from build123d import *

# Parameters (mm, degrees)
SKETCH_1_W                  = 180
SKETCH_1_H                  = 160
EXTRUDE_1_DEPTH             = 4
SKETCH_4_R                  = 1.6
CUT_EXTRUDE_3_DEPTH         = 4
SKETCH_5_R                  = 1.6
CUT_EXTRUDE_4_DEPTH         = 4
SKETCH_7_R                  = 2
CUT_EXTRUDE_5_DEPTH         = 10
FILLET_1_R                  = 10
SKETCH_8_R                  = 1.5
CUT_EXTRUDE_6_DEPTH         = 10
SKETCH_11_R                 = 1.5
CUT_EXTRUDE_8_DEPTH         = 4
SKETCH_12_R                 = 1.5
CUT_EXTRUDE_9_DEPTH         = 4
SKETCH_13_R                 = 1.5
CUT_EXTRUDE_10_DEPTH        = 10
PATTERN_LINEAR_1_COUNT      = 2
PATTERN_LINEAR_1_PITCH      = 30
PATTERN_LINEAR_1_COUNT_DIR2 = 2
PATTERN_LINEAR_1_PITCH_DIR2 = 30
MIRROR_1_COPY_1_SKETCH_R    = 1.5
MIRROR_1_COPY_1_DEPTH       = 10
MIRROR_1_COPY_2_SKETCH_R    = 1.5
MIRROR_1_COPY_2_DEPTH       = 10
MIRROR_1_COPY_3_SKETCH_R    = 1.5
MIRROR_1_COPY_3_DEPTH       = 10


with BuildPart() as part:
    # 草图1 → 凸台-拉伸1 (new body)
    with BuildSketch(Plane(origin=(0, 0, 0), x_dir=(1, 0, 0), z_dir=(0, 1, 0))):
        Rectangle(SKETCH_1_W, SKETCH_1_H)
    extrude(amount=EXTRUDE_1_DEPTH)

    # 草图4 → 切除-拉伸3 (cut)
    with BuildSketch(Plane(origin=(0, 4, 0), x_dir=(1, 0, 0), z_dir=(0, 1, 0))):
        with Locations(Location((-80, 56, 0), (0, 0, 270))):
            Circle(SKETCH_4_R)
        with Locations(Location((-43, 56, 0), (0, 0, 270))):
            Circle(SKETCH_4_R)
        with Locations(Location((-43, 19, 0), (0, 0, 270))):
            Circle(SKETCH_4_R)
        with Locations(Location((-80, 19, 0), (0, 0, 270))):
            Circle(SKETCH_4_R)
    extrude(amount=-CUT_EXTRUDE_3_DEPTH, mode=Mode.SUBTRACT)

    # 草图5 → 切除-拉伸4 (cut)
    with BuildSketch(Plane(origin=(0, 4, 0), x_dir=(1, 0, 0), z_dir=(0, 1, 0))):
        with Locations(Location((-78.7, -7.8, 0), (0, 0, 270))):
            Circle(SKETCH_5_R)
        with Locations(Location((-29.2, -23, 0), (0, 0, 270))):
            Circle(SKETCH_5_R)
        with Locations(Location((-29.2, -50.9, 0), (0, 0, 270))):
            Circle(SKETCH_5_R)
        with Locations(Location((-80, -56, 0), (0, 0, 270))):
            Circle(SKETCH_5_R)
        with Locations(Location((-29.2, -5.1, 0), (0, 0, 90))):
            Circle(SKETCH_5_R)
        with Locations(Location((-29.2, -33, 0), (0, 0, 90))):
            Circle(SKETCH_5_R)
        with Locations(Location((-80, 0, 0), (0, 0, 90))):
            Circle(SKETCH_5_R)
        with Locations(Location((-78.7, -48.2, 0), (0, 0, 90))):
            Circle(SKETCH_5_R)
    extrude(amount=-CUT_EXTRUDE_4_DEPTH, mode=Mode.SUBTRACT)

    # 草图7 → 切除-拉伸5 (cut)
    with BuildSketch(Plane.XZ):
        with Locations(Location((24, 35, 0), (0, 0, 270))):
            Circle(SKETCH_7_R)
        with Locations(Location((10, 35, 0), (0, 0, 270))):
            Circle(SKETCH_7_R)
        with Locations(Location((24, 3, 0), (0, 0, 270))):
            Circle(SKETCH_7_R)
        with Locations(Location((10, 3, 0), (0, 0, 270))):
            Circle(SKETCH_7_R)
    extrude(amount=-CUT_EXTRUDE_5_DEPTH, mode=Mode.SUBTRACT)

    # 圆角1
    fillet_1_edges = [part.edges().sort_by_distance(p)[0] for p in [
        (90, 2, 80),
        (-90, 2, 80),
        (-90, 2, -80),
        (90, 2, -80),
    ]]
    fillet(fillet_1_edges, radius=FILLET_1_R)

    # 草图8 → 切除-拉伸6 (cut)
    with BuildSketch(Plane.XZ):
        with Locations(Location((-14.949747468, 4.949747468, 0), (0, 0, 270))):
            Circle(SKETCH_8_R)
        with Locations(Location((-5.050252532, 4.949747468, 0), (0, 0, 270))):
            Circle(SKETCH_8_R)
        with Locations(Location((-14.949747468, -4.949747468, 0), (0, 0, 270))):
            Circle(SKETCH_8_R)
        with Locations(Location((-5.050252532, -4.949747468, 0), (0, 0, 270))):
            Circle(SKETCH_8_R)
    extrude(amount=-CUT_EXTRUDE_6_DEPTH, mode=Mode.SUBTRACT)

    # 草图11 → 切除-拉伸8 (cut)
    with BuildSketch(Plane.XZ):
        with Locations(Location((77, 12, 0), (0, 0, 270))):
            Circle(SKETCH_11_R)
        with Locations(Location((43, 12, 0), (0, 0, 90))):
            Circle(SKETCH_11_R)
        with Locations(Location((77, -12, 0), (0, 0, 90))):
            Circle(SKETCH_11_R)
        with Locations(Location((43, -12, 0), (0, 0, 270))):
            Circle(SKETCH_11_R)
    extrude(amount=-CUT_EXTRUDE_8_DEPTH, mode=Mode.SUBTRACT)

    # 草图12 → 切除-拉伸9 (cut)
    with BuildSketch(Plane.XZ):
        with Locations(Location((-86, 40, 0), (0, 0, 270))):
            Circle(SKETCH_12_R)
        with Locations(Location((-11, 40, 0), (0, 0, 270))):
            Circle(SKETCH_12_R)
        with Locations(Location((-11, -40, 0), (0, 0, 270))):
            Circle(SKETCH_12_R)
        with Locations(Location((-86, -40, 0), (0, 0, 270))):
            Circle(SKETCH_12_R)
    extrude(amount=-CUT_EXTRUDE_9_DEPTH, mode=Mode.SUBTRACT)

    # 草图13 → 切除-拉伸10 (cut)
    with BuildSketch(Plane(origin=(0, 4, 0), x_dir=(1, 0, 0), z_dir=(0, 1, 0))):
        with Locations(Location((80, 75, 0), (0, 0, 270))):
            Circle(SKETCH_13_R)
    cut_extrude_10 = extrude(amount=-CUT_EXTRUDE_10_DEPTH, mode=Mode.SUBTRACT)

    # 阵列(线性)1: Cut-Extrude 10 2 × 2
    with Locations(*[(-i * PATTERN_LINEAR_1_PITCH, 0, j * PATTERN_LINEAR_1_PITCH_DIR2) for i in range(PATTERN_LINEAR_1_COUNT) for j in range(PATTERN_LINEAR_1_COUNT_DIR2) if (i, j) != (0, 0)]):
        add(cut_extrude_10, mode=Mode.SUBTRACT)

    # 镜向1: 切除-拉伸10 across plane
    add(cut_extrude_10.mirror(Plane.XY), mode=Mode.SUBTRACT)

    # 镜向1 copy 1 sketch → 镜向1 copy 1 (cut)
    with BuildSketch(Plane(origin=(0, 4, -30), x_dir=(1, 0, 0), z_dir=(0, 1, 0))):
        with Locations((80, -75)):
            Circle(MIRROR_1_COPY_1_SKETCH_R)
    extrude(amount=-MIRROR_1_COPY_1_DEPTH, mode=Mode.SUBTRACT)

    # 镜向1 copy 2 sketch → 镜向1 copy 2 (cut)
    with BuildSketch(Plane(origin=(-30, 4, 0), x_dir=(1, 0, 0), z_dir=(0, 1, 0))):
        with Locations((80, -75)):
            Circle(MIRROR_1_COPY_2_SKETCH_R)
    extrude(amount=-MIRROR_1_COPY_2_DEPTH, mode=Mode.SUBTRACT)

    # 镜向1 copy 3 sketch → 镜向1 copy 3 (cut)
    with BuildSketch(Plane(origin=(-30, 4, -30), x_dir=(1, 0, 0), z_dir=(0, 1, 0))):
        with Locations((80, -75)):
            Circle(MIRROR_1_COPY_3_SKETCH_R)
    extrude(amount=-MIRROR_1_COPY_3_DEPTH, mode=Mode.SUBTRACT)


solid = part.part
Verification items for the finished model (mm, model axes). Round coordinates to 2 decimals unless told otherwise and drop trailing zeros. Put each result on its own line as item: value.
1) Material ranges on line 1 (X direction, y = 1.8, z = 40); line 2 (Z direction, x = 80, y = 2.1); line 3 (Z direction, x = -43.5, y = 1), recorded low to high.
Final values:
line 1: x = -90 to -87.5, -84.5 to -12.5, -9.5 to 90
line 2: z = -80 to -76.5, -73.5 to -46.5, -43.5 to 43.5, 46.5 to 73.5, 76.5 to 80
line 3: z = -80 to -57.52, -54.48 to -20.52, -17.48 to 80
2) Mould release check, pull along Z, two halves, no side actions. Record for faces 1 (the cylindrical face through (23.234, 1.972, 33.153)), 2 (the flat face through (90, 2, 1)), 3 (the cylindrical face through (-87.15, 2.03, 76.99)): +Z half, -Z half, draft (parallel to the pull), parting line (faces both ways), or undercut.
Final values:
face 1: undercut
face 2: draft
face 3: +Z half
3) Depth check by flat-ended pin: pin 1 (2.5 mm diameter, centred on x = 80, z = 45, fed in from -Y). Enter the tip coordinate at first touch or a pass-through.
Final values:
pin 1: passes through
